Build history of the part. All positions in model axes, mm. Face numbers are marked on the shaded views. A direction names the side the tool comes from. Give positions to 0.01 mm unless a question says otherwise; leave off trailing zeros. Order: outer loops, then holes, each group sorted by start corner. A loop starts at its lowest first (then second) coordinate and runs counter-clockwise, first axis right, second up. Notation, with made-up numbers: M 17.25,-12.5 L 24.25,-12.5 A10 ccw 24.25,0.5 Z; hole C -6.5,34.25 d4. An arc over 180 degrees is marked long. One line per item, written item: value.
from build123d import *

# Parameters (mm, degrees)
PAD018_DEPTH = 4
PAD019_DEPTH = 4
SKETCH035_R  = 2.5
PAD020_DEPTH = 4
PAD021_DEPTH = 4
PAD022_DEPTH = 4
SKETCH038_R  = 2.5
PAD023_DEPTH = 5
FILLET_R     = 2
FILLET001_R  = 2
FILLET002_R  = 4
FILLET003_R  = 4
SKETCH049_R  = 1.5
PAD028_DEPTH = 4


with BuildPart() as obj1:
    # Sketch033 → Pad018 (new body)
    with BuildSketch(Plane.XZ):
        with BuildLine():
            Line((44.945992765, 17.5), (110, 17.5))
            Line((110, 21.5), (110, 17.5))
            Line((44.1871982538, 21.5), (110, 21.5))
            ThreePointArc((42.6541143847, 20.8649758691), (43.3574992426, 21.3349626055), (44.1871982538, 21.5))
            Line((23.7891385155, 2), (42.6541143847, 20.8649758691))
            Line((0, 2), (23.7891385155, 2))
            ThreePointArc((0, -2), (-2, 0), (0, 2))
            Line((0, -2), (24.6175656403, -2))
            ThreePointArc((26.0317792027, -1.4142135624), (25.382932505, -1.847759065), (24.6175656403, -2))
            Line((26.0317792027, -1.4142135624), (44.945992765, 17.5))
        make_face()
    extrude(amount=-PAD018_DEPTH)

    # Sketch034 (on Face11 of Pad018) → Pad019 (join)
    with BuildSketch(Plane.XZ):
        with BuildLine():
            ThreePointArc((-5.64e-08, 5), (-5, -1.69e-08), (-2.26e-08, -5))
            Line((10.4599999543, -5), (-2.26e-08, -5))
            Line((14.8031457045, -0.6568542495), (10.4599999543, -5))
            Line((26.7891385155, -0.6568542495), (14.8031457045, -0.6568542495))
            Line((26.7891385155, 5), (26.7891385155, -0.6568542495))
            Line((26.7891385155, 5), (-5.64e-08, 5))
        make_face()
    extrude(amount=-PAD019_DEPTH)

    # Sketch035 (on Face13 of Pad019) → Pad020 (join)
    with BuildSketch(Plane.XZ):
        Circle(SKETCH035_R)
    extrude(amount=PAD020_DEPTH)

    # Sketch036 (on Face7 of Pad020) → Pad021 (join)
    with BuildSketch(Plane(origin=(0, 0, 21.5), x_dir=(-1, 0, 0), z_dir=(0, 0, 1))):
        Polygon((-110, 0), (-106, 0), (-106, -9), (-121.594421, -9), (-121.594421, -5), (-110, -5), align=None)
    extrude(amount=-PAD021_DEPTH)

    # Sketch037 (on Face12 of Pad021) → Pad022 (join)
    with BuildSketch(Plane(origin=(0, 9, 0), x_dir=(1, 0, 0), z_dir=(0, 1, 0))):
        with BuildLine():
            Line((121.594421, -21.5), (112.78511, -21.5))
            Line((112.78511, -21.5), (116.730789, -7.623817))
            ThreePointArc((124.6315830417, -11.7967375602), (122.1948418839, -6.844398802), (116.730789, -7.623817))
            Line((124.6315830417, -11.7967375602), (121.594421, -21.5))
        make_face()
    extrude(amount=-PAD022_DEPTH)

    # Sketch038 (on Face21 of Pad022) → Pad023 (join)
    with BuildSketch(Plane.XZ.offset(-5)):
        with Locations((120, 11)):
            Circle(SKETCH038_R)
    extrude(amount=PAD023_DEPTH)

    # Fillet
    fillet_edges = [obj1.edges().sort_by_distance(p)[0] for p in [
        (110, 0, 19.5),
        (106, 9, 19.5),
    ]]
    fillet(fillet_edges, radius=FILLET_R)

    # Fillet001
    fillet001_edges = [obj1.edges().sort_by_distance(p)[0] for p in [
        (106, 4, 19.5),
        (110, 5, 19.5),
    ]]
    fillet(fillet001_edges, radius=FILLET001_R)

    # Fillet002
    fillet002_edges = [obj1.edges().sort_by_distance(p)[0] for p in [
        (121.594421, 7, 21.5),
    ]]
    fillet(fillet002_edges, radius=FILLET002_R)

    # Fillet003
    fillet003_edges = [obj1.edges().sort_by_distance(p)[0] for p in [
        (26.789139, 2, 5),
        (10.46, 2, -5),
    ]]
    fillet(fillet003_edges, radius=FILLET003_R)

    # Sketch049 (on Face17 of Fillet003) → Pad028 (join)
    with BuildSketch(Plane(origin=(0, 4, 0), x_dir=(1, 0, 0), z_dir=(0, 1, 0))):
        with BuildLine():
            ThreePointArc((62, -13.5000013856), (58.0000006928, -9.5), (54, -13.5))
            Line((54, -13.5), (54, -17.5))
            Line((61.9999986144, -17.5), (54, -17.5))
            Line((62, -13.5000013856), (61.9999986144, -17.5))
        make_face()
        with Locations((58, -13.5)):
            Circle(SKETCH049_R, mode=Mode.SUBTRACT)
        with BuildLine():
            ThreePointArc((104, -13.5000013856), (100.0000006928, -9.5), (96, -13.5))
            Line((96, -13.5), (96, -17.5))
            Line((96, -17.5), (104, -17.5))
            Line((104, -17.5), (104, -13.5000013856))
        make_face()
        with Locations((100, -13.5)):
            Circle(SKETCH049_R, mode=Mode.SUBTRACT)
        with BuildLine():
            ThreePointArc((29.8256872599, -13.6934049535), (29.8256877498, -19.3502596929), (35.4825424892, -19.3502582232))
            Line((38.310969614, -16.5218310984), (35.4825424892, -19.3502582232))
            Line((32.6541153645, -10.8649768489), (38.310969614, -16.5218310984))
            Line((29.8256872599, -13.6934049535), (32.6541153645, -10.8649768489))
        make_face()
        with Locations((32.6541143847, -16.5218320782)):
            Circle(SKETCH049_R, mode=Mode.SUBTRACT)
    extrude(amount=-PAD028_DEPTH)


with BuildPart() as obj1_1:
    # Body004 placement: moved
    add(obj1.part.moved(Location((0, 8, 13))))


with BuildPart() as part_mirroring:
    # Part__Mirroring: instance of obj1
    add(obj1_1.part.mirror(Plane(origin=(0, 0, 0), x_dir=(1, 0, 0), z_dir=(0, 1, 0))))


with BuildPart() as part_mirroring_1:
    # Part__Mirroring placement: moved
    add(part_mirroring.part.moved(Location((9.2368815712, 50, 3.828366479))))


solid = part_mirroring_1.part
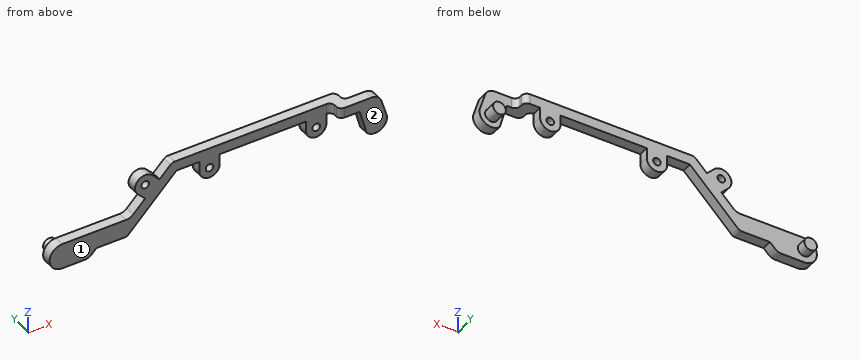
1) Saw through at B-B, the plane x = 74. Write the cut outline in (y, z).
Check values:
outline: M 38,34.33 L 42,34.33 L 42,38.33 L 38,38.33 Z
2) Pin check, flat tips, straight feed: pin 1 (1.2 mm diameter, centred on y = 41, z = 32, fed in from +X); pin 2 (4 mm diameter, centred on x = 109.24, z = 30.33, fed in from -Y); pin 3 (1.5 mm diameter, centred on x = 81, y = 43, fed in from -Z); pin 4 (4 mm diameter, centred on x = 125.5, z = 30, fed in from +Y). Stop position of each tip, or through.
Check values:
pin 1: x = 113.24
pin 2: y = 38
pin 3: through
pin 4: y = 42
3) Tool access for the marked faces 1 and 2: list every direction of +Z, -Z, +X, -X, +Y, -Y with a clear straight run to the whole face (end or side of a thin tool).
Check values:
face 1: +Z, -Z, -X, -Y
face 2: +Z, -Z, +X, -X, -Y
4) Drill centre lines: probe 1 along Y at (x, z) = (31, 15); probe 2 along X at (y, z) = (40, 34.25); probe 3 along X at (y, z) = (40.5, 25.75). Where is each one in solid material? Low to high. Write a range as from..to.
Check values:
probe 1: 38..42
probe 2: 37.99..40.69, 43.09..46.65, 48.45..54.1, 63.24..71.24, 105.24..113.24
probe 3: 39.95..45.6, 127.85..130.63
5) Saw through at A-A, the plane x = 109. Write the cut outline in (y, z), then the cut area to 3 significant figures.
Check values:
outline: M 38,26.34 L 42,26.34 L 42,28.85 L 38,28.85 Z; M 38,31.81 L 42,31.81 L 42,38.33 L 38,38.33 Z
area: 36.1 mm^2
